```python
from build123d import *

# Parameters (mm, degrees)
SKETCH1_R           = 12
BOSS_EXTRUDE1_DEPTH = 30.8
SKETCH2_R           = 12.5
BOSS_EXTRUDE2_DEPTH = 25
SKETCH3_R           = 3.5
BOSS_EXTRUDE3_DEPTH = 2.5
SKETCH6_R           = 11.75
BOSS_EXTRUDE5_DEPTH = 10.7
SKETCH7_W           = 18.699432978
SKETCH7_H           = 3
BOSS_EXTRUDE6_DEPTH = 20
SKETCH10_W          = 16.5
SKETCH10_H          = 1.5
CUT_EXTRUDE4_DEPTH  = 10
SKETCH4_R           = 2
CUT_EXTRUDE7_DEPTH  = 10
SKETCH11_R          = 1.5
SKETCH11_R_2        = 2
CUT_EXTRUDE8_DEPTH  = 10


with BuildPart() as part:
    # Sketch1 → Boss-Extrude1 (new body)
    with BuildSketch(Plane.XY):
        Circle(SKETCH1_R)
    extrude(amount=BOSS_EXTRUDE1_DEPTH)

    # Sketch2 → Boss-Extrude2 (add)
    with BuildSketch(Plane.XY.offset(30.8)):
        Circle(SKETCH2_R)
    extrude(amount=BOSS_EXTRUDE2_DEPTH)

    # Sketch3 → Boss-Extrude3 (add)
    with BuildSketch(Plane.XY.offset(55.8)):
        Circle(SKETCH3_R)
    extrude(amount=BOSS_EXTRUDE3_DEPTH)

    # Sketch6 → Boss-Extrude5 (add)
    with BuildSketch(Plane(origin=(0, 0, 0), x_dir=(-1, 0, 0), z_dir=(0, 0, -1))):
        Circle(SKETCH6_R)
    extrude(amount=BOSS_EXTRUDE5_DEPTH)

    # Sketch7 → Boss-Extrude6 (add)
    with BuildSketch(Plane(origin=(0, 0, 0), x_dir=(1, 0, 0), z_dir=(0, 1, 0))):
        with Locations((0, 6.81237414)):
            Rectangle(SKETCH7_W, SKETCH7_H)
    extrude(amount=BOSS_EXTRUDE6_DEPTH)

    # Sketch10 → Cut-Extrude4 (cut)
    with BuildSketch(Plane(origin=(0, 20, 0), x_dir=(1, 0, 0), z_dir=(0, 1, 0))):
        with Locations((0.137296408, 6.718389465)):
            Rectangle(SKETCH10_W, SKETCH10_H)
    extrude(amount=-CUT_EXTRUDE4_DEPTH, mode=Mode.SUBTRACT)

    # Sketch4 → Cut-Extrude7 (cut)
    with BuildSketch(Plane.XY.offset(58.3)):
        Circle(SKETCH4_R)
    extrude(amount=-CUT_EXTRUDE7_DEPTH, mode=Mode.SUBTRACT)

    # Sketch11 → Cut-Extrude8 (cut)
    with BuildSketch(Plane.XY.offset(55.8)):
        with Locations((0, 8.5)):
            Circle(SKETCH11_R)
        with Locations((8.5, 0)):
            Circle(SKETCH11_R_2)
        with Locations((-8.5, 0)):
            Circle(SKETCH11_R_2)
        with Locations((0, -8.5)):
            Circle(SKETCH11_R)
    extrude(amount=-CUT_EXTRUDE8_DEPTH, mode=Mode.SUBTRACT)


solid = part.part
```
Geometry: final body of the model. Coordinates: model frame, mm. A direction names the side the tool comes from. Give positions to 0.01 mm unless a question says otherwise; leave off trailing zeros. Loops run counter-clockwise (first coordinate to the right, second up) from the corner with the lowest first, then second, coordinate; pieces in that order, holes last. Notation, with made-up numbers: (-14, -34) - (31, -34) arc R16 cw to (31, -16) - close; hole circle Ø1 at (81, -14). An arc over 180 degrees is marked (long way). Answer as CSV lines item,"result". Start each with the question number.
(1) Section query B-B (z = 51). Output: boundary loops of the cut face in (x, y).
(2) Section query A-A (y = 0). Output: boundary loops of the cut face in (x, z), and give its area (3 significant figures).
(3) Section query C-C (x = -5.75). Output: boundary loops of the cut face in (y, z).
(4) Mould query, pull axis X, two halves, no side actions, for faces 1 (the face through (-7, 10, 30.8)), 2 (the face through (2.55, -11.47, -5.28)), 3 (the face through (0, 7, 51)). Classes: +X half, -X half, draft (parallel to the pull), parting line (faces both ways), or undercut.
(5) Section query D-D (y = 11). Output: boundary loops of the cut face in (x, z), and give its area (3 significant figures).
(6) Ray query, line 1 along Z through (x, y) = (3.25, 13); line 2 along Y through (x, z) = (0, 50); line 3 along X through (y, z) = (-1, 54). Return the intervals inside material, ascending. Write a range as [from, to].
(7) Pin query (flat end, axial travel): P1, Ø6, axis at y = 16, z = 6.5, coming from the -X side; P2, Ø6, axis at x = 5.5, z = 39, coming from the -Y side; P3, Ø1, axis at x = -8, z = 16, coming from the +Y side; P4, Ø1, axis at y = 8, z = 14.5, coming from the -X side. Return the tip coordinate at first contact, or that it passes through.
(8) Reachability of faces 4 (the face through (0, 9, 45.8)), 5 (the face through (-8.113, 15, -7)) from +Z, -Z, +X, -X, +Y, -Y: full face, straight path, thin tool, end or side. Return the list, or none.
Worked answers:
1,outline,"circle Ø25 at (0, 0); hole circle Ø4 at (-8.5, 0); hole circle Ø4 at (0, 0); hole circle Ø3 at (0, -8.5); hole circle Ø3 at (0, 8.5); hole circle Ø4 at (8.5, 0)"
2,outline,"(-12.5, 30.8) - (-12, 30.8) - (-12, 0) - (-11.75, 0) - (-11.75, -10.7) - (11.75, -10.7) - (11.75, 0) - (12, 0) - (12, 30.8) - (12.5, 30.8) - (12.5, 55.8) - (10.5, 55.8) - (10.5, 45.8) - (6.5, 45.8) - (6.5, 55.8) - (3.5, 55.8) - (3.5, 58.3) - (2, 58.3) - (2, 48.3) - (-2, 48.3) - (-2, 58.3) - (-3.5, 58.3) - (-3.5, 55.8) - (-6.5, 55.8) - (-6.5, 45.8) - (-10.5, 45.8) - (-10.5, 55.8) - (-12.5, 55.8) - close"
2,area,"1,510 mm^2"
3,outline,"(-11.1, 30.8) - (-10.53, 30.8) - (-10.53, 0) - (-10.25, 0) - (-10.25, -10.7) - (10.25, -10.7) - (10.25, -8.31) - (20, -8.31) - (20, -7.47) - (10, -7.47) - (10, -5.97) - (20, -5.97) - (20, -5.31) - (10.25, -5.31) - (10.25, 0) - (10.53, 0) - (10.53, 30.8) - (11.1, 30.8) - (11.1, 55.8) - (-11.1, 55.8) - close"
4,face 1,"draft"
4,face 2,"parting line"
4,face 3,"undercut"
5,outline,"(-9.35, -8.31) - (-4.13, -8.31) - (-4.13, -10.7) - (4.13, -10.7) - (4.13, -8.31) - (9.35, -8.31) - (9.35, -5.31) - (4.13, -5.31) - (4.13, 0) - (4.8, 0) - (4.8, 30.8) - (5.94, 30.8) - (5.94, 55.8) - (-5.94, 55.8) - (-5.94, 30.8) - (-4.8, 30.8) - (-4.8, 0) - (-4.13, 0) - (-4.13, -5.31) - (-9.35, -5.31) - close; hole (-8.11, -7.47) - (8.39, -7.47) - (8.39, -5.97) - (-8.11, -5.97) - close"
5,area,"687 mm^2"
6,line 1,"z = [-8.31, -7.47], [-5.97, -5.31]"
6,line 2,"y = [-12.5, -10], [-7, -2], [2, 7], [10, 12.5]"
6,line 3,"x = [-12.46, -10.23], [-6.77, -1.73], [1.73, 6.77], [10.23, 12.46]"
7,P1,"passes through"
7,P2,"stops at y = -12.25"
7,P3,"stops at y = 9.37"
7,P4,"stops at x = -9.37"
8,face 4,"+Z"
8,face 5,"+Y"
